Source: three-view drawing plus pictorial views. Frame: mm from the lowest corner of the part. A direction names the side the tool comes from. Give positions to 0.01 mm unless a question says otherwise; leave off trailing zeros. Loops run counter-clockwise (first coordinate to the right, second up) from the corner with the lowest first, then second, coordinate; pieces in that order, holes last. Notation, with made-up numbers: M 76,-20.5 L 115,-20.5 A32 cw 115,9.5 Z; hole C 62.25,58 d1. An arc over 180 degrees is marked long. One line per item, written item: value. Start each with the question number.
(1) Access query for the marked faces 5, 6 and 7. Directions: +Z, -Z, +X, -X, +Y, -Y. A direction counts if a zero-diameter tool reaches every point of the face in a straight line with its end or side. Return the directions, or none.
(2) Pin query (flat end, axial travel): P1, Ø12.5, axis at x = 34, y = 42.5, coming from the +Z side; P2, Ø24, axis at x = 78, z = 53, coming from the +Y side; P3, Ø7.5, axis at x = 63.5, y = 14, coming from the +Z side. Return the tip coordinate at first contact, or that it passes through.
(3) Pull-direction query (X, two-part tool) for the marked faces 1, 2, 3 and 4; classes: released by +X, released by -X, zero draft, split by the parting line, or undercut.
(4) Section B-B on y = 34. Output: boundary loops of the cut face in (x, z), plus the area to 3 significant figures.
(5) Section D-D on z = 59. Output: boundary loops of the cut face in (x, y), plus the area to 3 significant figures.
(6) Section C-C on x = 55. Output: boundary loops of the cut face in (y, z), plus the area to 3 significant figures.
(7) Section A-A on z = 12.5. Output: boundary loops of the cut face in (x, y).
(8) Ray query, line 1 along X through (y, z) = (18, 12); line 2 along Y through (x, z) = (104.5, 50.5). Return the intervals inside material, ascending. Write a range as from..to.
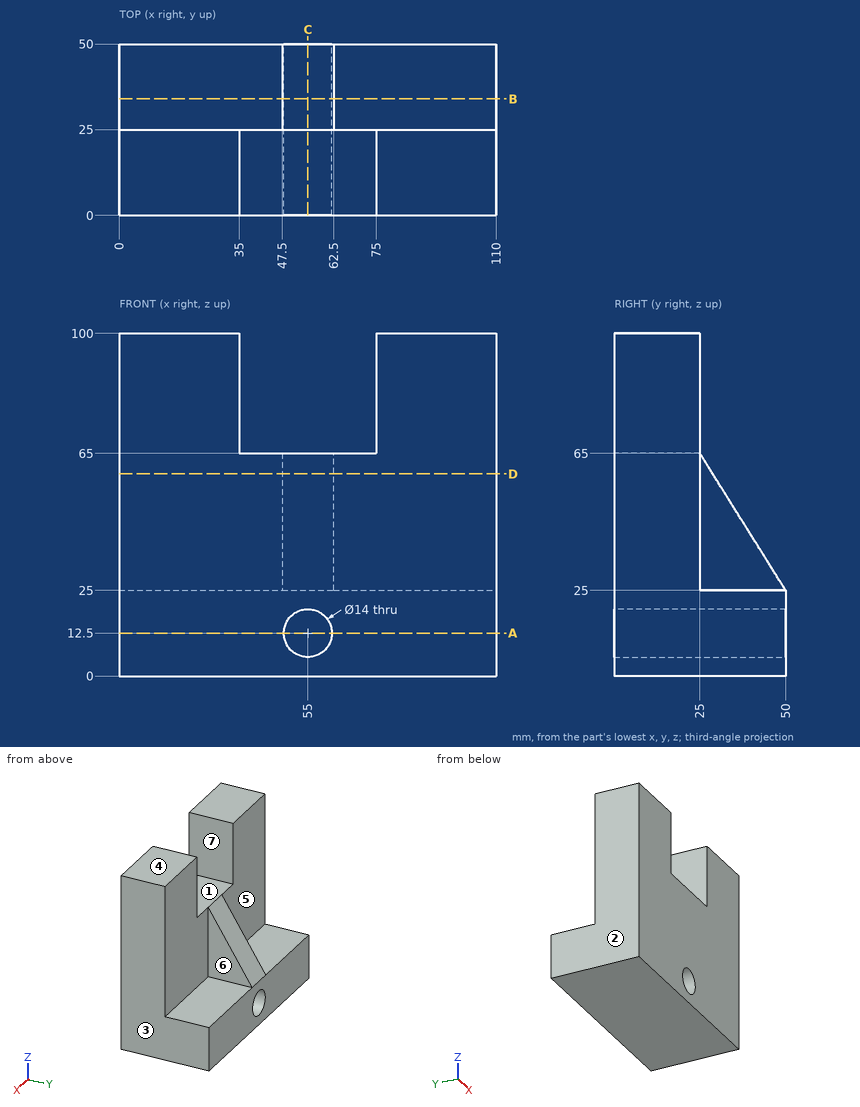
Output values:
1. face 5: +Z, -X, +Y
1. face 6: +Z, +X, +Y
1. face 7: +Z, +Y, -Y
2. P1: stops at z = 25
2. P2: stops at y = 25
2. P3: stops at z = 65
3. face 1: undercut
3. face 2: released by -X
3. face 3: released by +X
3. face 4: zero draft
4. outline: M 0,0 L 110,0 L 110,25 L 62.5,25 L 62.5,50.6 L 47.5,50.6 L 47.5,25 L 0,25 Z; hole C 55,12.5 d14
4. area: 2,980 mm²
5. outline: M 0,0 L 110,0 L 110,25 L 62.5,25 L 62.5,28.75 L 47.5,28.75 L 47.5,25 L 0,25 Z
5. area: 2,810 mm²
6. outline: M 0,0 L 50,0 L 50,5.5 L 0,5.5 Z; M 0,19.5 L 50,19.5 L 50,25 L 25,65 L 0,65 Z
6. area: 2,050 mm²
7. outline: M 0,0 L 48,0 L 48,50 L 0,50 Z; M 62,0 L 110,0 L 110,50 L 62,50 Z
8. line 1: x = 0..48.02, 61.98..110
8. line 2: y = 0..25
